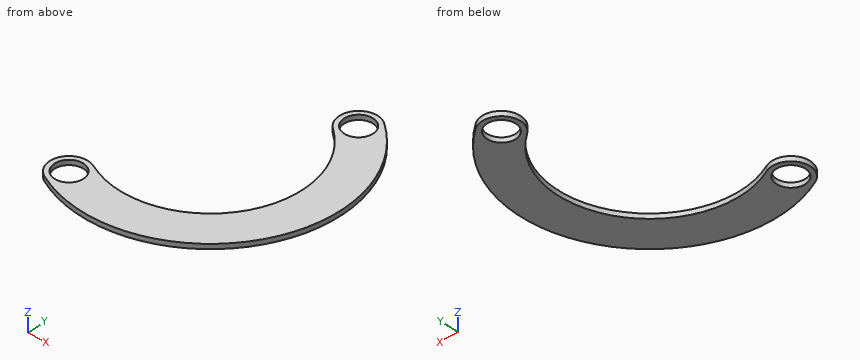
```python
from build123d import *

# Parameters (mm, degrees)
ESQUISSE1_R               = 3
T_LE_DE_BASE_PLI_E1_DEPTH = 1


# Sheet-metal steps are written as plain solids
with BuildPart() as part:
    # Esquisse1 → Tôle de base pliée1 (new body)
    with BuildSketch(Plane.XY):
        with BuildLine():
            ThreePointArc((-33.586634848, -37.422563624), (1.75063467, -27.854557121), (-4.720147653, 8.178737781))
            ThreePointArc((-4.720147653, 8.178737781), (-10.326052384, 7.421220682), (-9.568535285, 1.815315952))
            ThreePointArc((-9.568535285, 1.815315952), (-5.008878396, -23.575657367), (-29.909395263, -30.317782906))
            ThreePointArc((-29.909395263, -30.317782906), (-35.300405414, -32.031553473), (-33.586634848, -37.422563624))
        make_face()
        with Locations((-31.748015055, -33.870173265)):
            Circle(ESQUISSE1_R, mode=Mode.SUBTRACT)
        with Locations((-7.144341469, 4.997026867)):
            Circle(ESQUISSE1_R, mode=Mode.SUBTRACT)
    extrude(amount=-T_LE_DE_BASE_PLI_E1_DEPTH)


solid = part.part
```
Work out the finished part from the listing and answer in its coordinate system (mm). Coordinates: 2 decimals unless noted, no trailing zeros. Loops run counter-clockwise (first coordinate to the right, second up) from the corner with the lowest first, then second, coordinate; pieces in that order, holes last.
1) Section B-B (x = -6) is taken. Give the vertices of the cut face in (y, z), plus the area to 3 significant figures.
Results:
outline: (-35.83, -1) - (-24.99, -1) - (-24.99, 0) - (-35.83, 0) - close; (-1.74, -1) - (2.22, -1) - (2.22, 0) - (-1.74, 0) - close; (7.77, -1) - (8.83, -1) - (8.83, 0) - (7.77, 0) - close
area: 15.9 mm2
2) Section C-C (z = -0.8) is taken. Give the vertices of the cut face in (x, y), plus the area to 3 significant figures.
Results:
outline: (-33.59, -37.42) arc R27.09 ccw to (-4.72, 8.18) arc R4 ccw to (-9.57, 1.82) arc R19.09 cw to (-29.91, -30.32) arc R4 ccw to start; hole circle Ø6 at (-31.75, -33.87); hole circle Ø6 at (-7.14, 5)
area: 542 mm2
3) Flat-ended cylindrical pins translate along their axes: pin 1 (10 mm diameter, centred on x = -11, y = -29.5, fed in from +Z); pin 2 (3.5 mm diameter, centred on x = -7.14, y = 5, fed in from -Z). Find the tip coordinate at first contact, or state that the pin passes through.
Results:
pin 1: stops at z = 0
pin 2: passes through
4) Consider probe 1 along Y at (x, z) = (-30.5, -0.2); probe 2 along X at (y, z) = (4, -0.5); probe 3 along Y at (x, z) = (-34, -0.8). Determine where each line is inside the solid, lowest interval first.
Results:
probe 1: y = -38.78 to -36.6, -31.14 to -30.07
probe 2: x = -11.02 to -9.97, -4.31 to -0.35
probe 3: y = -37.18 to -35.85, -31.89 to -30.56
5) Section D-D (y = -28) is taken. Give the vertices of the cut face in (x, z), plus the area to 3 significant figures.
Results:
outline: (-8.88, -1) - (1.66, -1) - (1.66, 0) - (-8.88, 0) - close
area: 10.5 mm2
6) Section A-A (y = -36) is taken. Give the vertices of the cut face in (x, z).
Results:
outline: (-35.13, -1) - (-33.86, -1) - (-33.86, 0) - (-35.13, 0) - close; (-29.64, -1) - (-6.26, -1) - (-6.26, 0) - (-29.64, 0) - close
